from build123d import *

# Parameters (mm, degrees)
SKETCH_1_R      = 1.75
SKETCH_1_R_2    = 5
SKETCH_1_R_3    = 1.6
EXTRUDE_1_DEPTH = 2.5


with BuildPart() as part:
    # 草图1 → 凸台-拉伸1 (new body)
    with BuildSketch(Plane(origin=(0, 0, 0), x_dir=(1, 0, 0), z_dir=(0, 1, 0))):
        with BuildLine():
            ThreePointArc((-61, -29.99135156), (-58.071067812, -37.062419372), (-51, -39.99135156))
            Line((-51, -39.99135156), (51, -39.99135156))
            ThreePointArc((51, -39.99135156), (58.071067812, -37.062419372), (61, -29.99135156))
            Line((61, -29.99135156), (61, 22.277696204))
            add(Edge.make_bspline(
                [(61, 22.277696204), (62.293823386, 26.079256197), (56.634308682, 31.150713443), (52.485620359, 36.687772359), (52, 40.715903778)],
                knots=[0, 0, 0, 0, 0.462697284, 1, 1, 1, 1], degree=3))
            Line((52, 40.715903778), (52, 58.880539276))
            add(Edge.make_bspline(
                [(52, 58.880539276), (51.906435238, 66.324037), (48.17922794, 79.056777751), (37.094065188, 85.955470032), (37, 91.294061848)],
                knots=[0, 0, 0, 0, 0.617360936, 1, 1, 1, 1], degree=3))
            Line((37, 91.294061848), (37, 104.845172054))
            ThreePointArc((37, 104.845172054), (35.535533906, 108.38070596), (32, 109.845172054))
            Line((32, 109.845172054), (-32, 109.845172054))
            ThreePointArc((-32, 109.845172054), (-35.535533906, 108.38070596), (-37, 104.845172054))
            Line((-37, 104.845172054), (-37, 91.294061848))
            add(Edge.make_bspline(
                [(-52, 58.880539276), (-51.906435238, 66.324037), (-48.17922794, 79.056777751), (-37.094065188, 85.955470032), (-37, 91.294061848)],
                knots=[0, 0, 0, 0, 0.617360936, 1, 1, 1, 1], degree=3))
            Line((-52, 58.880539276), (-52, 40.715903778))
            add(Edge.make_bspline(
                [(-61, 22.277696204), (-62.293823386, 26.079256197), (-56.634308682, 31.150713443), (-52.485620359, 36.687772359), (-52, 40.715903778)],
                knots=[0, 0, 0, 0, 0.462697284, 1, 1, 1, 1], degree=3))
            Line((-61, 22.277696204), (-61, -29.99135156))
        make_face()
        with Locations(Location((-53, -8.5, 0), (0, 0, 270))):
            Circle(SKETCH_1_R, mode=Mode.SUBTRACT)
        with Locations(Location((-44.5, 0, 0), (0, 0, 270))):
            Circle(SKETCH_1_R_2, mode=Mode.SUBTRACT)
        with Locations(Location((-36, -8.5, 0), (0, 0, 270))):
            Circle(SKETCH_1_R, mode=Mode.SUBTRACT)
        with Locations(Location((-53, 8.5, 0), (0, 0, 270))):
            Circle(SKETCH_1_R, mode=Mode.SUBTRACT)
        with Locations(Location((-36, 8.5, 0), (0, 0, 270))):
            Circle(SKETCH_1_R, mode=Mode.SUBTRACT)
        with BuildLine():
            ThreePointArc((-41.5, 18.25), (-43.13586607, 19.88586607), (-41.5, 21.52173214))
            Line((-41.5, 21.52173214), (-6.629379417, 21.52173214))
            ThreePointArc((-6.629379417, 21.52173214), (-4.993513347, 19.88586607), (-6.629379417, 18.25))
            Line((-6.629379417, 18.25), (-41.5, 18.25))
        make_face(mode=Mode.SUBTRACT)
        with BuildLine():
            ThreePointArc((-41.5, 27.1), (-43.13586607, 28.73586607), (-41.5, 30.37173214))
            Line((-41.5, 30.37173214), (-6.629379417, 30.37173214))
            ThreePointArc((-6.629379417, 30.37173214), (-4.993513347, 28.73586607), (-6.629379417, 27.1))
            Line((-6.629379417, 27.1), (-41.5, 27.1))
        make_face(mode=Mode.SUBTRACT)
        with BuildLine():
            ThreePointArc((-41.5, 35.95), (-43.13586607, 37.58586607), (-41.5, 39.22173214))
            Line((-41.5, 39.22173214), (-6.629379417, 39.22173214))
            ThreePointArc((-6.629379417, 39.22173214), (-4.993513347, 37.58586607), (-6.629379417, 35.95))
            Line((-6.629379417, 35.95), (-41.5, 35.95))
        make_face(mode=Mode.SUBTRACT)
        with BuildLine():
            ThreePointArc((-41.5, 44.8), (-43.13586607, 46.43586607), (-41.5, 48.07173214))
            Line((-41.5, 48.07173214), (-6.629379417, 48.07173214))
            ThreePointArc((-6.629379417, 48.07173214), (-4.993513347, 46.43586607), (-6.629379417, 44.8))
            Line((-6.629379417, 44.8), (-41.5, 44.8))
        make_face(mode=Mode.SUBTRACT)
        with Locations(Location((36, -8.5, 0), (0, 0, 270))):
            Circle(SKETCH_1_R, mode=Mode.SUBTRACT)
        with Locations(Location((53, -8.5, 0), (0, 0, 270))):
            Circle(SKETCH_1_R, mode=Mode.SUBTRACT)
        with Locations(Location((44.5, 0, 0), (0, 0, 270))):
            Circle(SKETCH_1_R_2, mode=Mode.SUBTRACT)
        with Locations(Location((36, 8.5, 0), (0, 0, 270))):
            Circle(SKETCH_1_R, mode=Mode.SUBTRACT)
        with Locations(Location((53, 8.5, 0), (0, 0, 270))):
            Circle(SKETCH_1_R, mode=Mode.SUBTRACT)
        with BuildLine():
            Line((6.629379417, 21.52173214), (41.5, 21.52173214))
            ThreePointArc((41.5, 21.52173214), (43.13586607, 19.88586607), (41.5, 18.25))
            Line((41.5, 18.25), (6.629379417, 18.25))
            ThreePointArc((6.629379417, 18.25), (4.993513347, 19.88586607), (6.629379417, 21.52173214))
        make_face(mode=Mode.SUBTRACT)
        with BuildLine():
            Line((6.629379417, 30.37173214), (41.5, 30.37173214))
            ThreePointArc((41.5, 30.37173214), (43.13586607, 28.73586607), (41.5, 27.1))
            Line((41.5, 27.1), (6.629379417, 27.1))
            ThreePointArc((6.629379417, 27.1), (4.993513347, 28.73586607), (6.629379417, 30.37173214))
        make_face(mode=Mode.SUBTRACT)
        with BuildLine():
            Line((6.629379417, 39.22173214), (41.5, 39.22173214))
            ThreePointArc((41.5, 39.22173214), (43.13586607, 37.58586607), (41.5, 35.95))
            Line((41.5, 35.95), (6.629379417, 35.95))
            ThreePointArc((6.629379417, 35.95), (4.993513347, 37.58586607), (6.629379417, 39.22173214))
        make_face(mode=Mode.SUBTRACT)
        with BuildLine():
            Line((6.629379417, 48.07173214), (41.5, 48.07173214))
            ThreePointArc((41.5, 48.07173214), (43.13586607, 46.43586607), (41.5, 44.8))
            Line((41.5, 44.8), (6.629379417, 44.8))
            ThreePointArc((6.629379417, 44.8), (4.993513347, 46.43586607), (6.629379417, 48.07173214))
        make_face(mode=Mode.SUBTRACT)
        with BuildLine():
            ThreePointArc((-48.931385346, 53.73119276), (-50.581385346, 55.38119276), (-48.931385346, 57.03119276))
            Line((-48.931385346, 57.03119276), (-24.064689708, 57.03119276))
            ThreePointArc((-24.064689708, 57.03119276), (-22.414689708, 55.38119276), (-24.064689708, 53.73119276))
            Line((-24.064689708, 53.73119276), (-48.931385346, 53.73119276))
        make_face(mode=Mode.SUBTRACT)
        with BuildLine():
            Line((-47.365035435, 65.58311996), (-27.274768907, 65.58311996))
            ThreePointArc((-27.274768907, 65.58311996), (-25.624768907, 63.93311996), (-27.274768907, 62.28311996))
            Line((-27.274768907, 62.28311996), (-47.365035435, 62.28311996))
            ThreePointArc((-47.365035435, 62.28311996), (-49.015035435, 63.93311996), (-47.365035435, 65.58311996))
        make_face(mode=Mode.SUBTRACT)
        with BuildLine():
            Line((-44.932457044, 73.982304528), (-28.97899618, 73.982304528))
            ThreePointArc((-28.97899618, 73.982304528), (-27.32899618, 72.332304528), (-28.97899618, 70.682304528))
            Line((-28.97899618, 70.682304528), (-44.932457044, 70.682304528))
            ThreePointArc((-44.932457044, 70.682304528), (-46.582457044, 72.332304528), (-44.932457044, 73.982304528))
        make_face(mode=Mode.SUBTRACT)
        with Locations(Location((-21.145483371, 79.821873209, 0), (0, 0, 270))):
            Circle(SKETCH_1_R_3, mode=Mode.SUBTRACT)
        with BuildLine():
            Line((32, 105.037777769), (0, 105.037777769))
            Line((0, 105.037777769), (-32, 105.037777769))
            ThreePointArc((-32, 105.037777769), (-33.65, 106.687777769), (-32, 108.337777769))
            Line((-32, 108.337777769), (32, 108.337777769))
            ThreePointArc((32, 108.337777769), (33.65, 106.687777769), (32, 105.037777769))
        make_face(mode=Mode.SUBTRACT)
        with BuildLine():
            Line((24.064689708, 57.03119276), (48.931385346, 57.03119276))
            ThreePointArc((48.931385346, 57.03119276), (50.581385346, 55.38119276), (48.931385346, 53.73119276))
            Line((48.931385346, 53.73119276), (24.064689708, 53.73119276))
            ThreePointArc((24.064689708, 53.73119276), (22.414689708, 55.38119276), (24.064689708, 57.03119276))
        make_face(mode=Mode.SUBTRACT)
        with BuildLine():
            Line((27.274768907, 65.58311996), (47.365035435, 65.58311996))
            ThreePointArc((47.365035435, 65.58311996), (49.015035435, 63.93311996), (47.365035435, 62.28311996))
            Line((47.365035435, 62.28311996), (27.274768907, 62.28311996))
            ThreePointArc((27.274768907, 62.28311996), (25.624768907, 63.93311996), (27.274768907, 65.58311996))
        make_face(mode=Mode.SUBTRACT)
        with BuildLine():
            Line((44.932457044, 70.682304528), (28.97899618, 70.682304528))
            ThreePointArc((28.97899618, 70.682304528), (27.32899618, 72.332304528), (28.97899618, 73.982304528))
            Line((28.97899618, 73.982304528), (44.932457044, 73.982304528))
            ThreePointArc((44.932457044, 73.982304528), (46.582457044, 72.332304528), (44.932457044, 70.682304528))
        make_face(mode=Mode.SUBTRACT)
        with BuildLine():
            ThreePointArc((0, 62.821873209), (-17, 79.821873209), (0, 96.821873209))
            ThreePointArc((0, 96.821873209), (17, 79.821873209), (0, 62.821873209))
        make_face(mode=Mode.SUBTRACT)
        with Locations(Location((21.145483371, 79.821873209, 0), (0, 0, 270))):
            Circle(SKETCH_1_R_3, mode=Mode.SUBTRACT)
    extrude(amount=EXTRUDE_1_DEPTH)


solid = part.part
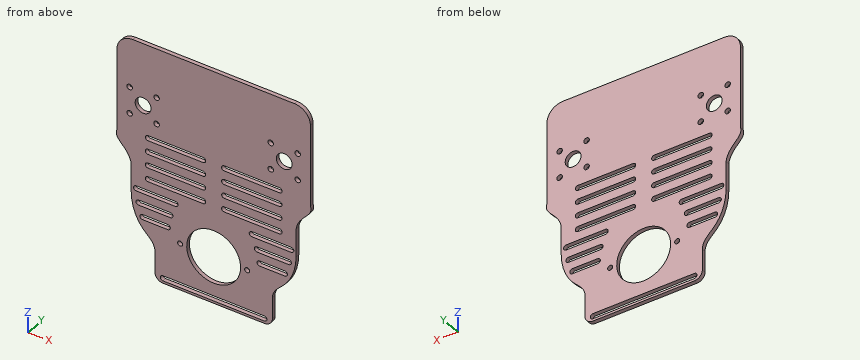
Model file for the job. Use its own axes, mm. Give positions to 0.01 mm unless a question says otherwise; leave off trailing zeros. Write each loop counter-clockwise with the first axis right and the second up, starting at its lowest first coordinate (ties: lowest second). Pieces come first, ordered by that corner, then holes. Notation, with made-up numbers: (4, 83.25) - (35, 83.25) arc R18 cw to (35, 118.25) - close; hole circle Ø7 at (-33.75, 12.5). An arc over 180 degrees is marked (long way). Answer as CSV lines item,"result".
1. Pin check, flat tips, straight feed: pin 1 (4 mm diameter, centred on x = 36, z = -8.5, fed in from +Y); pin 2 (1.2 mm diameter, centred on y = 0.5, z = -98, fed in from +X); pin 3 (1 mm diameter, centred on x = 49, y = 1.5, fed in from -Z). Stop position of each tip, or through.
Responses:
pin 1,"stops at y = 2.5"
pin 2,"stops at x = 37"
pin 3,"stops at z = -73.93"
2. Band-saw the part on A-A (z = 0). Write the cut outline in (x, y).
Responses:
outline,"(-61, 0) - (-49.5, 0) - (-49.5, 2.5) - (-61, 2.5) - close; (-39.5, 0) - (39.5, 0) - (39.5, 2.5) - (-39.5, 2.5) - close; (49.5, 0) - (61, 0) - (61, 2.5) - (49.5, 2.5) - close"
3. Band-saw the part on D-D (z = -50). Write the cut outline in (x, y), and give its area (3 significant figures).
Responses:
outline,"(-52, 0) - (52, 0) - (52, 2.5) - (-52, 2.5) - close"
area,"260 mm2"
4. Band-saw the part on B-B (x = 0). Write the cut outline in (y, z), and give its area (3 significant figures).
Responses:
outline,"(0, -109.85) - (2.5, -109.85) - (2.5, -108.34) - (0, -108.34) - close; (0, -105.04) - (2.5, -105.04) - (2.5, -96.82) - (0, -96.82) - close; (0, -62.82) - (2.5, -62.82) - (2.5, 39.99) - (0, 39.99) - close"
area,"281 mm2"
5. Drill centre lines: L1, parallel to X at y = 1.2, z = 0; L2, parallel to Z at x = -18, y = 2.2; L3, parallel to X at y = 0.95, z = -8.5. Where is each one in solid material? Low to high. Write a range as [from, to].
Responses:
L1,"x = [-61, -49.5], [-39.5, 39.5], [49.5, 61]"
L2,"z = [-109.85, -108.34], [-105.04, -48.07], [-44.8, -39.22], [-35.95, -30.37], [-27.1, -21.52], [-18.25, 39.99]"
L3,"x = [-61, -54.75], [-51.25, -37.75], [-34.25, 34.25], [37.75, 51.25], [54.75, 61]"
6. Band-saw the part on C-C (y = 1.05). Count the separate pieces of the cut face and the enclosed holes in it, and give its area (3 significant figures).
Responses:
separate pieces,"1"
enclosed holes,"28"
area,"13,100 mm2"
